Check sheet for the modelled part. Datum: model origin and axes. Units: mm. Give positions to 0.01 mm unless a question says otherwise; leave off trailing zeros. Loops run counter-clockwise (first coordinate to the right, second up) from the corner with the lowest first, then second, coordinate; pieces in that order, holes last. Notation, with made-up numbers: (-35.75, 18.5) -> (-27.75, 18.5) arc R32 cw to (-27.75, 56.5) -> close; hole circle Ø11 at (18, 51). An arc over 180 degrees is marked (long way). Write each question's results on one line, items separated by ' | '. Start each with the question number.
Item 1: Cross-section at A-A on z = 204.5. Enter the section's corners in (x, y), then the cut area to 3 significant figures.
Item 2: Scan lines: line 1 along Z through (x, y) = (-4.35, 0); line 2 along Z through (x, y) = (-0.25, 4.5); line 3 along X through (y, z) = (3.5, 82). Record each from-to range of solid material in increasing order.
Item 3: Cross-section at B-B on x = 0. State how many separate pieces and enclosed holes the cut face has, then the cut area to 3 significant figures.
Autodesk Inventor part; units mm, degrees
ref_plane "YZ Plane" through (0, 0, 0) normal (1, 0, 0) x (0, 1, 0)
ref_plane "XZ Plane" through (0, 0, 0) normal (0, 1, 0) x (-1, 0, 0)
ref_plane "XY Plane" through (0, 0, 0) normal (0, 0, 1) x (1, 0, 0)
sketch "スケッチ1" plane through (0, 0, 0) normal (0, 0, 1) x (1, 0, 0)
  line L0 (5, -5) -> (-5, -5)
  line L1 (-5, -5) -> (-5, 5)
  line L2 (-5, 5) -> (5, 5)
  line L3 (5, 5) -> (5, -5)
  line L4 (5, -5) -> (-5, 5) construction
  line L5 (-5, -5) -> (5, 5) construction
  line L6 (4, 4) -> (-4, 4)
  line L7 (-4, 4) -> (-4, -4)
  line L8 (-4, -4) -> (4, -4)
  line L9 (4, -4) -> (4, 4)
  point P0 (0, 0)
  dimension "d0" = 10
  dimension "d1" = 10
  dimension "d2" = 1
extrude "押し出し1" add sketch "スケッチ1" along normal blind 300
sketch "スケッチ2" plane through (5, -5, 0) normal (1, 0, 0) x (0, 0, -1)
  line L0 (0, 0) -> (0, 10)
  line L1 (0, 10) -> (-300, 10)
  line L2 (-300, 0) -> (-300, 10)
  line L3 (0, 0) -> (-300, 0)
  line L4 (0, 5) -> (-300, 5)
  line L5 (-300, 0) -> (-300, 10)
  point P0 (-290, 5)
  point P1 (-182, 5)
  point P2 (-62, 5)
  point P3 (-10, 5)
  point P4 (-118, 5)
  dimension "d7" = 120
  dimension "d25" = 10
  dimension "d26" = 52
  dimension "d27" = 10
  dimension "d28" = 108
  dimension "d29" = 56
hole "穴1" at (5, 0, 290) at (5, 0, 182) at (5, 0, 62) at (5, 0, 10) at (5, 0, 118) direction (-1, 0, 0) diameter 3.3 end through all
sketch "スケッチ3" plane through (-5, 5, 0) normal (0, 1, 0) x (1, 0, 0)
  line L0 (10, 0) -> (0, 0)
  line L1 (0, 0) -> (0, -300)
  line L2 (10, -300) -> (0, -300)
  line L3 (10, 0) -> (10, -300)
  line L4 (5, -300) -> (5, 0)
  point P0 (5, -275)
  point P1 (5, -52)
  point P2 (5, -108)
  point P3 (5, -192)
  point P4 (5, -25)
  dimension "d17" = 25
  dimension "d30" = 52
  dimension "d31" = 56
  dimension "d32" = 84
  dimension "d33" = 25
hole "穴2" at (0, 5, 275) at (0, 5, 52) at (0, 5, 108) at (0, 5, 192) at (0, 5, 25) direction (0, -1, 0) diameter 3.3 end through all
properties part number "kaku_1010_200"
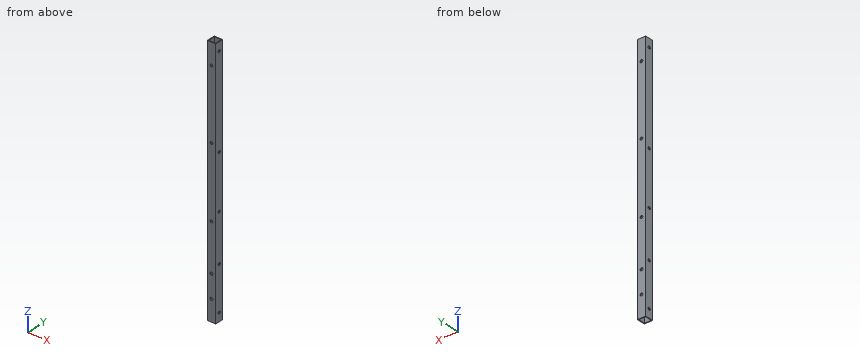
Answer sheet:
1) outline: (-5, -5) -> (5, -5) -> (5, 5) -> (-5, 5) -> close; hole (-4, -4) -> (4, -4) -> (4, 4) -> (-4, 4) -> close | area: 36.0 mm²
2) line 1: z = 0 to 8.35, 11.65 to 60.35, 63.65 to 116.35, 119.65 to 180.35, 183.65 to 288.35, 291.65 to 300 | line 2: z = 0 to 23.37, 26.63 to 50.37, 53.63 to 106.37, 109.63 to 190.37, 193.63 to 273.37, 276.63 to 300 | line 3: x = -5 to -4, 4 to 5
3) separate pieces: 12 | enclosed holes: 0 | area: 567 mm²
